Could you check a few things on this model? Use its own coordinates, in mm. A direction names the side the tool comes from. Give positions to 0.01 mm unless a question says otherwise; leave off trailing zeros. Order: outer loops, then holes, each group sorted by start corner. A loop starts at its lowest first (then second) coordinate and runs counter-clockwise, first axis right, second up. Notation, with made-up numbers: (54.25, -6) - (82.25, -6) arc R15 cw to (82.25, -2) - close; hole circle Ø3 at (-3.5, 40). An arc over 180 degrees is marked (long way). One line per question, with ' | ' between items. Start each with the question number.
1. Imagine slicing it at C-C (x = 77). Please give me the cut outline in (y, z).
2. Imagine slicing it at A-A (y = 5). Please give me the cut outline in (x, z).
3. Imagine slicing it at D-D (y = 42). Please give me the cut outline in (x, z), and give its area (3 significant figures).
4. Which directions (+Z, -Z, +X, -X, +Y, -Y) give clear straight access to the entire face, cutting with the end or side of a thin tool? Please do faces 4 (the flat face through (158.4, 10, 7.2)), 5 (the flat face through (80, 72, 9)), 6 (the flat face through (158, 5, 6)), 7 (the flat face through (1.6, 62, 7.2)).
5. For P1, Ø5, axis at x = 5.5, z = 5, coming from the -Y side; P2, Ø1, axis at y = 25, z = 9, coming from the -X side; P3, Ø4, axis at x = 39, y = 14.5, coming from the -Z side; P4, Ø2, axis at y = 28.5, z = 8.5, coming from the +X side, each with a flat end and sliding along its axis, tell me the tip position at first contact or that it passes through.
6. If we mould it in two halves opening along X, with no side actions, what happens to faces 1 (the flat face through (158.4, 62, 7.2)), 2 (the flat face through (160, 67, 6)), 3 (the flat face through (79, 37, 8))? For each: released by +X, released by -X, zero draft, split by the parting line, or undercut.
7. I need wall thicknesses on probe 1 along Z at (x, y) = (0.5, 67); probe 2 along X at (y, z) = (68, 7); probe 3 along Z at (x, y) = (140.5, 30). Which ranges of each line are inside material? Lowest first, please. Write a range as from..to.
8. Imagine slicing it at B-B (z = 4). Give the number of separate pieces and of enclosed holes in the cut face, and give its area (3 significant figures).
```python
from build123d import *

# Parameters (mm, degrees)
BOX002_W     = 156
BOX002_H     = 72
BOX002_DEPTH = 8
BOX001_W     = 10
BOX001_H     = 52
BOX001_DEPTH = 10
BOX_W        = 160
BOX_H        = 72
BOX_DEPTH    = 10
SKETCH_R     = 1.65
HOLE_DEPTH   = 160.001


with BuildPart() as obj1:
    # Box002 → Box002 (new body)
    with BuildSketch(Plane(origin=(2, 0, 0), x_dir=(1, 0, 0), z_dir=(0, 0, 1))):
        with Locations((78, 36)):
            Rectangle(BOX002_W, BOX002_H)
    extrude(amount=BOX002_DEPTH)


with BuildPart() as obj2:
    # Box001 → Box001 (new body)
    with BuildSketch(Plane(origin=(0, 10, 0), x_dir=(1, 0, 0), z_dir=(0, 0, 1))):
        with Locations((5, 26)):
            Rectangle(BOX001_W, BOX001_H)
    extrude(amount=BOX001_DEPTH)


with BuildPart() as part_mirroring:
    # Part__Mirroring: instance of obj2
    add(obj2.part.mirror(Plane(origin=(80, 0, 0), x_dir=(0, -1, 0), z_dir=(1, 0, 0))))


with BuildPart() as body:
    # Box → Box (new body)
    with BuildSketch(Plane.XY):
        with Locations((80, 36)):
            Rectangle(BOX_W, BOX_H)
    extrude(amount=BOX_DEPTH)

    # Cut: cut obj2
    add(obj2.part, mode=Mode.SUBTRACT)

    # Cut001: cut Part__Mirroring
    add(part_mirroring.part, mode=Mode.SUBTRACT)

    # Cut002: cut obj1
    add(obj1.part, mode=Mode.SUBTRACT)

    # Sketch (on Face1 of BaseFeature) → Hole (cut, through all)
    with BuildSketch(Plane(origin=(0, 0, 0), x_dir=(0, -1, 0), z_dir=(-1, 0, 0))):
        with Locations((-5, 4)):
            Circle(SKETCH_R)
        with Locations((-67, 4)):
            Circle(SKETCH_R)
    extrude(amount=-HOLE_DEPTH, mode=Mode.SUBTRACT)


solid = body.part
```
Results found:
1) outline: (0, 8) - (72, 8) - (72, 10) - (0, 10) - close
2) outline: (0, 0) - (2, 0) - (2, 2.35) - (0, 2.35) - close; (0, 5.65) - (2, 5.65) - (2, 8) - (158, 8) - (158, 5.65) - (160, 5.65) - (160, 10) - (0, 10) - close; (158, 0) - (160, 0) - (160, 2.35) - (158, 2.35) - close
3) outline: (10, 8) - (150, 8) - (150, 10) - (10, 10) - close | area: 280 mm2
4) face 4: +Z, -Z, +X | face 5: +Z, -Z, +X, -X, +Y | face 6: -Z, +Y, -Y | face 7: +Z, -Z, -X
5) P1: passes through | P2: stops at x = 10 | P3: stops at z = 8 | P4: stops at x = 150
6) face 1: zero draft | face 2: released by +X | face 3: undercut
7) probe 1: z = 0..2.35, 5.65..10 | probe 2: x = 0..2, 158..160 | probe 3: z = 8..10
8) separate pieces: 8 | enclosed holes: 0 | area: 53.6 mm2
